```python
from build123d import *

# Parameters (mm, degrees)
BOSS_EXTRUDE1_DEPTH = 15.3
SKETCH2_R           = 2.3
CUT_EXTRUDE1_DEPTH  = 16.3
SKETCH3_R           = 16.25
SKETCH3_R_2         = 11.65
CUT_EXTRUDE2_DEPTH  = 10
SKETCH4_W           = 16.4
SKETCH4_H           = 12.7
CUT_EXTRUDE3_DEPTH  = 5
CUT_EXTRUDE6_DEPTH  = 1
CUT_EXTRUDE7_DEPTH  = 0.5


with BuildPart() as part:
    # Sketch1 → Boss-Extrude1 (new body)
    with BuildSketch(Plane(origin=(0, 0, 0), x_dir=(1, 0, 0), z_dir=(0, 1, 0))):
        with BuildLine():
            Line((0, 0), (0, 19))
            Line((0, 19), (26.7, 19))
            ThreePointArc((26.7, 19), (32.797644088, 17.95548785), (38.2, 14.941052635))
            ThreePointArc((38.2, 14.941052635), (40.271433107, 14.311273646), (42.2, 15.295187477))
            Line((42.2, 15.295187477), (43.269443579, 16.525441584))
            ThreePointArc((43.269443579, 16.525441584), (48.087218379, 16.862333216), (48.424110012, 12.044558416))
            Line((48.424110012, 12.044558416), (47.354666433, 10.814304309))
            ThreePointArc((47.354666433, 10.814304309), (46.801667822, 9.415462269), (47.248710238, 7.979245156))
            ThreePointArc((47.248710238, 7.979245156), (45.289416111, -24.409093359), (13.030186992, -27.899858595))
            ThreePointArc((13.030186992, -27.899858595), (12.183303759, -27.710109359), (11.432636129, -28.14567117))
            Line((11.432636129, -28.14567117), (10.187606856, -29.710887484))
            ThreePointArc((10.187606856, -29.710887484), (5.389112516, -30.257606856), (4.842393144, -25.459112516))
            Line((4.842393144, -25.459112516), (6.087422418, -23.893896202))
            ThreePointArc((6.087422418, -23.893896202), (7.124082388, -21.152735596), (6.372856996, -18.320018566))
            ThreePointArc((6.372856996, -18.320018566), (3.237759838, -10.229166003), (3.5, -1.556106595))
            ThreePointArc((3.5, -1.556106595), (2.927161914, -0.445774177), (1.76, 0))
            Line((1.76, 0), (0, 0))
        make_face()
    extrude(amount=BOSS_EXTRUDE1_DEPTH)

    # Sketch2 → Cut-Extrude1 (cut, through all)
    with BuildSketch(Plane(origin=(0, 15.3, 0), x_dir=(1, 0, 0), z_dir=(0, 1, 0))):
        with Locations((45.846776795, 14.285)):
            Circle(SKETCH2_R)
        with Locations((7.515, -27.585)):
            Circle(SKETCH2_R)
    extrude(amount=-CUT_EXTRUDE1_DEPTH, mode=Mode.SUBTRACT)

    # Sketch3 → Cut-Extrude2 (cut)
    with BuildSketch(Plane(origin=(0, 15.3, 0), x_dir=(1, 0, 0), z_dir=(0, 1, 0))):
        with Locations((27.093039229, -7.054893275)):
            Circle(SKETCH3_R)
        with Locations((27.093039229, -7.054893275)):
            Circle(SKETCH3_R_2, mode=Mode.SUBTRACT)
    extrude(amount=-CUT_EXTRUDE2_DEPTH, mode=Mode.SUBTRACT)

    # Sketch4 → Cut-Extrude3 (cut)
    with BuildSketch(Plane.ZY):
        with Locations((-9.5, 7.65)):
            Rectangle(SKETCH4_W, SKETCH4_H)
    extrude(amount=-CUT_EXTRUDE3_DEPTH, mode=Mode.SUBTRACT)

    # Sketch5 → Cut-Extrude6 (cut)
    with BuildSketch(Plane.XZ):
        Polygon((24.473039229, 32.3), (24.473039229, 22.4), (29.713039229, 22.4), (29.713039229, 30.3), (25.773039229, 30.3), (25.773039229, 31.6), (29.713039229, 31.6), (29.713039229, 32.3), align=None)
    extrude(amount=-CUT_EXTRUDE6_DEPTH, mode=Mode.SUBTRACT)

    # Sketch6 → Cut-Extrude7 (cut)
    with BuildSketch(Plane.XZ):
        with BuildLine():
            ThreePointArc((20.446034334, 16.982126203), (28.294472835, 19.55144458), (35.841272267, 16.198057911))
            Line((35.841272267, 16.198057911), (43.97300025, 24.329785894))
            ThreePointArc((43.97300025, 24.329785894), (35.608102686, 29.66755154), (25.773039229, 30.984662069))
            Line((25.773039229, 30.984662069), (25.773039229, 30.3))
            Line((25.773039229, 30.3), (29.713039229, 30.3))
            Line((29.713039229, 30.3), (29.713039229, 22.4))
            Line((29.713039229, 22.4), (24.473039229, 22.4))
            Line((24.473039229, 22.4), (24.473039229, 30.837474717))
            ThreePointArc((24.473039229, 30.837474717), (17.69194169, 28.770137265), (11.862557451, 24.735853266))
            Line((11.862557451, 24.735853266), (20.446034334, 16.982126203))
        make_face()
        with BuildLine():
            ThreePointArc((16.242880644, 8.941329927), (17.141710334, 12.601843748), (19.175813557, 15.775119708))
            Line((19.175813557, 15.775119708), (10.642082831, 23.48390949))
            ThreePointArc((10.642082831, 23.48390949), (6.404884497, 16.733017379), (4.726194331, 8.941329927))
            Line((4.726194331, 8.941329927), (16.242880644, 8.941329927))
        make_face()
        with BuildLine():
            ThreePointArc((18.982670233, 0.576892744), (17.084929659, 3.665470455), (16.242880644, 7.191329927))
            Line((16.242880644, 7.191329927), (4.726194331, 7.191329927))
            ThreePointArc((4.726194331, 7.191329927), (6.460315035, -0.735389017), (10.839143244, -7.566634245))
            Line((10.839143244, -7.566634245), (18.982670233, 0.576892744))
        make_face()
        with BuildLine():
            ThreePointArc((25.962402252, -3.30017766), (22.906366669, -2.382568809), (20.2201071, -0.660544123))
            Line((20.2201071, -0.660544123), (12.076580111, -8.804071112))
            ThreePointArc((12.076580111, -8.804071112), (18.505879136, -13.011918289), (25.962402252, -14.867215257))
            Line((25.962402252, -14.867215257), (25.962402252, -3.30017766))
        make_face()
        with BuildLine():
            Line((43.342508455, -8.804071112), (35.198981466, -0.660544123))
            ThreePointArc((35.198981466, -0.660544123), (31.702722743, -2.718127676), (27.709544283, -3.433670073))
            Line((27.709544283, -3.433670073), (27.709544283, -14.933670073))
            ThreePointArc((27.709544283, -14.933670073), (36.105399692, -13.346507623), (43.342508455, -8.804071112))
        make_face()
        with BuildLine():
            Line((50.692894235, 7.191329927), (39.176207922, 7.191329927))
            ThreePointArc((39.176207922, 7.191329927), (38.334158907, 3.665470455), (36.436418333, 0.576892744))
            Line((36.436418333, 0.576892744), (44.579945322, -7.566634245))
            ThreePointArc((44.579945322, -7.566634245), (48.958773531, -0.735389017), (50.692894235, 7.191329927))
        make_face()
        with BuildLine():
            Line((45.161425577, 23.047379266), (36.982294854, 14.868248542))
            ThreePointArc((36.982294854, 14.868248542), (38.494390898, 12.058457617), (39.176207922, 8.941329927))
            Line((39.176207922, 8.941329927), (50.692894235, 8.941329927))
            ThreePointArc((50.692894235, 8.941329927), (49.122090569, 16.462928139), (45.161425577, 23.047379266))
        make_face()
    extrude(amount=-CUT_EXTRUDE7_DEPTH, mode=Mode.SUBTRACT)


solid = part.part
```
Model file for the job. Use its own axes, mm. A direction names the side the tool comes from. Round coordinates to 2 decimals unless told otherwise and drop trailing zeros. Loops run counter-clockwise (first coordinate to the right, second up) from the corner with the lowest first, then second, coordinate; pieces in that order, holes last. Notation, with made-up numbers: M -3,-22 L 10,-22 A30 cw 10,7 Z; hole C -20,-33 d1. An arc over 180 degrees is marked long. Put each result on its own line as item: value. Start each with the question number.
Item 1: Cut at A-A (y = 8.75). Give the number of separate pieces and of enclosed holes in the cut face, then the cut area to 3 significant figures.
Item 2: Drill centre lines: line 1 along Z through (x, y) = (33.5, 13.5); line 2 along X through (y, z) = (12.75, -15.5); line 3 along Z through (x, y) = (31.5, 9.5). Where is each one in solid material? Low to high.
Item 3: Mould opens along Z. For faces 5 (the face through (2.94, 7.54, 0.46)), 6 (the face through (13, 8, -19)), 7 (the face through (12.196, 7.543, 27.708)) say: released by +Z, released by -Z, zero draft, split by the parting line, or undercut.
Item 4: Cut at D-D (x = 32). List the corners of the cut face in (y, z), then the cut area to 3 significant figures.
Item 5: 3-axis set-ups, long thin cutter, end or side, ignore diameter. For faces 1 (the face through (40.451, 0.246, -3.438)), 2 (the face through (27, 15.3, 7)), 3 (the face through (2, 8, -1.3)), 4 (the face through (38.205, 10.37, 3.556)): which of +Z, -Z, +X, -X, +Y, -Y reach the whole face in a straight line?
Item 6: Drop flat-ended pins along their axis: P1, Ø3, axis at y = 2.5, z = 19, coming from the +X side; P2, Ø2, axis at x = 23.5, z = -5.5, coming from the -Y side; P3, Ø0.6, axis at x = 27.5, y = 0.5, coming from the -Z side. Give the stop position or say it passes through.
Item 7: Cut at C-C (y = 4.5). List the corners of the cut face in (x, z) (1 decimal).
Item 8: Cut at B-B (z = 12). List the corners of the cut face in (x, y).
Answer block:
1. separate pieces: 2
1. enclosed holes: 3
1. area: 1,720 mm2
2. line 1: -17.69 to -7.88, -2.68 to 16.78, 21.99 to 31.37
2. line 2: 5 to 37.47, 42.38 to 43.89, 47.8 to 49.04
2. line 3: -18.36 to -8.59, -3.73 to 17.84, 22.7 to 31.81
3. face 5: undercut
3. face 6: released by -Z
3. face 7: released by +Z
4. outline: M 0,-18.22 L 15.3,-18.22 L 15.3,-8.44 L 5.3,-8.44 L 5.3,-3.51 L 15.3,-3.51 L 15.3,17.62 L 5.3,17.62 L 5.3,22.55 L 15.3,22.55 L 15.3,31.72 L 0,31.72 L 0,30.66 L 0.5,30.66 L 0.5,18.74 L 0,18.74 L 0,-2.6 L 0.5,-2.6 L 0.5,-14.53 L 0,-14.53 Z
4. area: 654 mm2
5. face 1: -Y
5. face 2: +Z, -Z, +X, -X, +Y
5. face 3: -X
5. face 4: +Y
6. P1: x = 49.97
6. P2: y = 0.5
6. P3: z = -18.99
7. outline: M 0,-19 L 26.7,-19 A18.3 ccw 38.2,-14.9 A2.9 cw 42.2,-15.3 L 43.3,-16.5 A3.4 ccw 48.4,-12 L 47.4,-10.8 A2.3 cw 47.2,-8 A25.1 ccw 13,27.9 A1.2 cw 11.4,28.1 L 10.2,29.7 A3.4 ccw 4.8,25.5 L 6.1,23.9 A4.8 cw 6.4,18.3 A21.8 ccw 3.5,1.6 A1.8 cw 1.8,0 L 0,0 L 0,-1.3 L 5,-1.3 L 5,-17.7 L 0,-17.7 Z; hole C 7.5,27.6 d4.6; hole C 45.8,-14.3 d4.6
8. outline: M 3.62,0 L 5.05,0 L 5.05,0.5 L 16.9,0.5 L 16.9,0 L 38.52,0 L 38.52,0.5 L 50.37,0.5 L 50.37,0 L 51.75,0 L 51.75,15.3 L 42.57,15.3 L 42.57,5.3 L 37.64,5.3 L 37.64,15.3 L 16.54,15.3 L 16.54,5.3 L 11.61,5.3 L 11.61,15.3 L 3.62,15.3 Z
